Geometry check sheet. Reference: the model listing, model coordinates, mm. A direction names the side the tool comes from. Round coordinates to 2 decimals unless told otherwise and drop trailing zeros. Order: outer loops, then holes, each group sorted by start corner. A loop starts at its lowest first (then second) coordinate and runs counter-clockwise, first axis right, second up. Notation, with made-up numbers: (39, -25.5) - (58, -25.5) arc R21 cw to (58, -0.5) - close; hole circle Ø1 at (11.5, 75). An arc over 180 degrees is marked (long way). Write each question's results on one line, items separated by ' | '.
```python
from build123d import *

# Parameters (mm, degrees)
ESQUISSE1_R        = 2.2
BOSS_EXTRU_1_DEPTH = 10


with BuildPart() as part:
    # Esquisse1 → Boss.-Extru.1 (new body)
    with BuildSketch(Plane(origin=(0, 0, 0), x_dir=(1, 0, 0), z_dir=(0, 1, 0))):
        with BuildLine():
            Line((0.042215238, -149.99999406), (-8.86714291, -108.577292103))
            Line((-8.86714291, -108.577292103), (52.724318579, -95.32995759))
            Line((52.724318579, -95.32995759), (61.633676726, -136.752659547))
            ThreePointArc((61.633676726, -136.752659547), (75, -129.903810568), (87.61443884, -121.752659547))
            ThreePointArc((87.61443884, -121.752659547), (91.272869966, -29.412659164), (142.217130056, 47.689494845))
            ThreePointArc((142.217130056, 47.689494845), (136.735308263, 61.672161259), (129.882697804, 75.036556498))
            Line((129.882697804, 75.036556498), (98.46426469, 46.609475032))
            Line((98.46426469, 46.609475032), (56.196005726, 93.325578082))
            Line((56.196005726, 93.325578082), (87.61443884, 121.752659547))
            ThreePointArc((87.61443884, 121.752659547), (75, 129.903810568), (61.633676726, 136.752659547))
            ThreePointArc((61.633676726, 136.752659547), (-20.164324954, 93.750953649), (-112.408879058, 99.318900059))
            ThreePointArc((-112.408879058, 99.318900059), (-121.777312488, 87.58016992), (-129.924913042, 74.963437562))
            Line((-129.924913042, 74.963437562), (-89.59712178, 61.96781707))
            Line((-89.59712178, 61.96781707), (-108.920324304, 2.004379509))
            Line((-108.920324304, 2.004379509), (-149.248115566, 15))
            ThreePointArc((-149.248115566, 15), (-150, 0), (-149.248115566, -15))
            ThreePointArc((-149.248115566, -15), (-71.108545012, -64.338294485), (-29.808250998, -147.008394905))
            ThreePointArc((-29.808250998, -147.008394905), (-14.957995775, -149.252331179), (0.042215238, -149.99999406))
        make_face()
        with Locations(Location((-5.571030795, -45.433447067, 0), (0, 0, 270))):
            Circle(ESQUISSE1_R, mode=Mode.SUBTRACT)
        with Locations(Location((0.663417157, -74.419562014, 0), (0, 0, 270))):
            Circle(ESQUISSE1_R, mode=Mode.SUBTRACT)
        with Locations(Location((29.992684533, -68.111307484, 0), (0, 0, 90))):
            Circle(ESQUISSE1_R, mode=Mode.SUBTRACT)
        with Locations(Location((23.758236581, -39.125192537, 0), (0, 0, 90))):
            Circle(ESQUISSE1_R, mode=Mode.SUBTRACT)
        with Locations(Location((41.871759308, 17.656574754, 0), (0, 0, 270))):
            Circle(ESQUISSE1_R, mode=Mode.SUBTRACT)
        with Locations(Location((64.117522664, 37.784317118, 0), (0, 0, 270))):
            Circle(ESQUISSE1_R, mode=Mode.SUBTRACT)
        with Locations(Location((43.9897803, 60.030080475, 0), (0, 0, 90))):
            Circle(ESQUISSE1_R, mode=Mode.SUBTRACT)
        with Locations(Location((21.744016943, 39.902338111, 0), (0, 0, 90))):
            Circle(ESQUISSE1_R, mode=Mode.SUBTRACT)
        with Locations(Location((-36.226921935, 27.433719884, 0), (0, 0, 270))):
            Circle(ESQUISSE1_R, mode=Mode.SUBTRACT)
        with Locations(Location((-64.780939821, 36.635244896, 0), (0, 0, 270))):
            Circle(ESQUISSE1_R, mode=Mode.SUBTRACT)
        with Locations(Location((-73.982464833, 8.081227009, 0), (0, 0, 90))):
            Circle(ESQUISSE1_R, mode=Mode.SUBTRACT)
        with Locations(Location((-45.428446946, -1.120298002, 0), (0, 0, 90))):
            Circle(ESQUISSE1_R, mode=Mode.SUBTRACT)
    extrude(amount=BOSS_EXTRU_1_DEPTH)


solid = part.part
```
(1) Material ranges on line 1 (X direction, y = 7.25, z = -38.5); line 2 (Z direction, x = 42, y = 7.25); line 3 (Z direction, x = -116, y = 1.5), recorded low to high.
Answers follow:
line 1: -97.16 to -65.95, -63.61 to 20.05, 23.44 to 62.04, 66.2 to 132.43 | line 2: -120.79 to -60.97, -59.09 to -19.85, -15.46 to 97.64 | line 3: -95.1 to -70.48, -4.29 to 28.9
(2) Draft check along X on faces 6 (the face through (-128.8, 4.93, -8.41)), 7 (the face through (77.626, 4.93, -69.641)), 8 (the face through (75.18, 4.93, -129.8)), 9 (the face through (-71.99, 4.93, 63.37)). Enter one of: released by +X, released by -X, zero draft, split by the parting line, or undercut.
Answers follow:
face 6: undercut | face 7: undercut | face 8: released by +X | face 9: released by -X
(3) Section check D-D (z = 10). Record the cut outline in (x, y).
Answers follow:
outline: (-149.67, 0) - (98.86, 0) - (98.86, 10) - (-149.67, 10) - close
(4) Section check B-B (x = 78). Record the cut outline in (y, z).
Answers follow:
outline: (0, -128.12) - (10, -128.12) - (10, -113.05) - (0, -113.05) - close; (0, -69.23) - (10, -69.23) - (10, 128.12) - (0, 128.12) - close
(5) Access from +Z, -Z, +X, -X, +Y, -Y to the whole of each face (thin tool, end or side, straight path). Record for faces 1 (the face through (-110.043, 4.93, -68.557)), 2 (the face through (57.117, 4.93, 115.751)), 3 (the face through (114.39, 4.93, -61.02)), 4 (the face through (-4.35, 4.93, 129.58)), 5 (the face through (71.685, 4.93, -107.34)).
Answers follow:
face 1: -X, +Y, -Y | face 2: +Z, +Y, -Y | face 3: -Z, +Y, -Y | face 4: +Y, -Y | face 5: +X, +Y, -Y
(6) Section check C-C (y = 3.5). Give the number of separate pieces and of enclosed holes in the cut face, then the cut area to 3 significant figures.
Answers follow:
separate pieces: 1 | enclosed holes: 12 | area: 42,500 mm²
(7) Section check A-A (z = -71.5). Record the cut outline in (x, y).
Answers follow:
outline: (-119.18, 0) - (75.94, 0) - (75.94, 10) - (-119.18, 10) - close; (125.97, 0) - (131.86, 0) - (131.86, 10) - (125.97, 10) - close
(8) Depth check by flat-ended pin: pin 1 Ø2.5 at (x, z) = (-64.78, -36.64) entering from +Y; pin 2 Ø3 at (x, y) = (-97, 9) entering from -Z; pin 3 Ø3 at (x, y) = (42, 2) entering from +Z; pin 4 Ø1.5 at (y, z) = (3, 68.5) entering from -X. Enter the tip coordinate at first touch or a pass-through.
Answers follow:
pin 1: through | pin 2: z = -95.17 | pin 3: z = 97.96 | pin 4: x = -68.1
